Part model, mm, in its own coordinate system. Round coordinates to 2 decimals unless told otherwise and drop trailing zeros. Write each loop counter-clockwise with the first axis right and the second up, starting at its lowest first coordinate (ties: lowest second). Pieces come first, ordered by that corner, then holes.
1) Flat gauge pins, fed straight in: pin 1 (4 mm diameter, centred on y = 16.5, z = 9.5, fed in from -X); pin 2 (2 mm diameter, centred on x = 8.5, y = 7.5, fed in from -Z); pin 3 (1 mm diameter, centred on y = 16, z = 13.5, fed in from +X); pin 4 (1 mm diameter, centred on x = 4.5, y = 18, fed in from -Z). Where does each tip first touch, or does it go through?
2) Saw through at B-B on z = 14.75. Write the cut outline in (x, y), and give its area (3 significant figures).
3) Drill centre lines: L1, parallel to X at y = 19, z = 2.5; L2, parallel to Z at x = 18.75, y = 19.25; L3, parallel to Z at x = 7.25, y = 12.5. Where is each one in solid material? Low to high.
4) Saw through at C-C on x = 12. Write the cut outline in (y, z).
5) Saw through at A-A on y = 15.25. Write the cut outline in (x, z).
```python
from build123d import *

# Parameters (mm, degrees)
SKETCH1_W           = 20
SKETCH1_H           = 20
BOSS_EXTRUDE1_DEPTH = 20
CUT_EXTRUDE1_DEPTH  = 20
CUT_EXTRUDE2_DEPTH  = 20


with BuildPart() as part:
    # Sketch1 → Boss-Extrude1 (new body)
    with BuildSketch(Plane.XY):
        with Locations((10, 10)):
            Rectangle(SKETCH1_W, SKETCH1_H)
    extrude(amount=BOSS_EXTRUDE1_DEPTH)

    # Sketch2 → Cut-Extrude1 (cut)
    with BuildSketch(Plane(origin=(0, 20, 0), x_dir=(1, 0, 0), z_dir=(0, 1, 0))):
        Polygon((20, -20), (20, -10), (10, -20), align=None)
    extrude(amount=-CUT_EXTRUDE1_DEPTH, mode=Mode.SUBTRACT)

    # Sketch3 → Cut-Extrude2 (cut)
    with BuildSketch(Plane(origin=(0, 20, 0), x_dir=(1, 0, 0), z_dir=(0, 1, 0))):
        Polygon((0, 0), (10, 0), (0, -10), align=None)
    extrude(amount=-CUT_EXTRUDE2_DEPTH, mode=Mode.SUBTRACT)


solid = part.part
```
Completed:
1. pin 1: stops at x = 0
1. pin 2: stops at z = 0.5
1. pin 3: stops at x = 17
1. pin 4: stops at z = 5
2. outline: (0, 0) - (15.25, 0) - (15.25, 20) - (0, 20) - close
2. area: 305 mm2
3. L1: x = 7.5 to 20
3. L2: z = 0 to 11.25
3. L3: z = 2.75 to 20
4. outline: (0, 0) - (20, 0) - (20, 18) - (0, 18) - close
5. outline: (0, 10) - (10, 0) - (20, 0) - (20, 10) - (10, 20) - (0, 20) - close
